The model under review builds one solid part; all positions refer to its coordinate system, in mm. Give positions to 0.01 mm unless a question says otherwise; leave off trailing zeros. Loops run counter-clockwise (first coordinate to the right, second up) from the corner with the lowest first, then second, coordinate; pieces in that order, holes last. Notation, with made-up numbers: M -5.75,-39 L 30.25,-39 A15 ccw 30.25,-35 Z; hole C -29,70 d3. An arc over 180 degrees is marked long. Put each result on its own line as item: value. Start each with the question number.
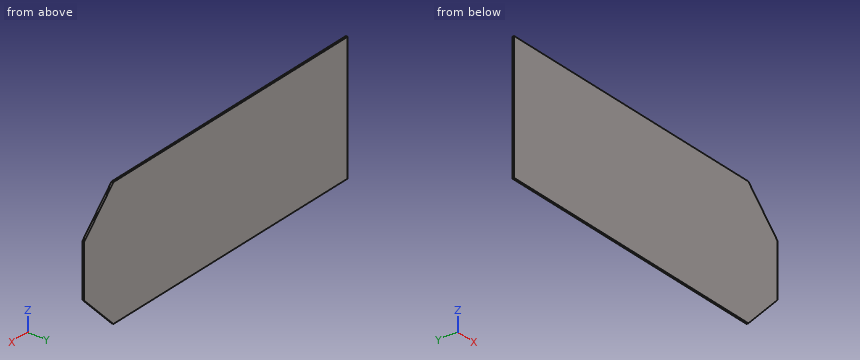
Autodesk Inventor part; units mm, degrees
ref_plane "YZ Plane" through (0, 0, 0) normal (1, 0, 0) x (0, 1, 0)
ref_plane "XZ Plane" through (0, 0, 0) normal (0, 1, 0) x (-1, 0, 0)
ref_plane "XY Plane" through (0, 0, 0) normal (0, 0, 1) x (1, 0, 0)
sketch "Sketch1" plane through (0, 0, 0) normal (0, 1, 0) x (-1, 0, 0)
  line L0 (-60.5593, 27.4889) -> (62.6411, -28.4339) construction
  line L1 (62.6424, 27.1286) -> (-64.3576, -27.8714) construction
  line L2 (-77.4954, -16.5) -> (-44.4954, -16.5) construction
  line L3 (-63.5, 27.7812) -> (63.5, 27.7812)
  line L4 (63.5, 27.7812) -> (63.5, -27.7812)
  line L5 (63.5, -27.7812) -> (-63.5, -27.7812)
  line L6 (-63.5, 27.7812) -> (63.5, -27.7812) construction
  line L7 (63.5, 27.7812) -> (-63.5, -27.7812) construction
  line L8 (-63.5, 11.5094) -> (63.5, 11.5094)
  line L9 (63.5, 11.5094) -> (63.5, -11.5094)
  line L10 (63.5, -11.5094) -> (-63.5, -11.5094)
  line L11 (-63.5, 11.5094) -> (63.5, -11.5094) construction
  line L12 (63.5, 11.5094) -> (-63.5, -11.5094) construction
  line L13 (-79.375, 11.5094) -> (-79.375, -11.5094)
  line L14 (-63.5, 27.7812) -> (-79.375, 11.5094)
  line L15 (-79.375, -11.5094) -> (-63.5, -27.7812)
  point P0 (0, 0)
  dimension "d1" = 55.5625
  dimension "d6" = 127
  dimension "d7" = 55.5625
  dimension "d8" = 127
  dimension "d9" = 23.0188
extrude "Extrusion1" add sketch "Sketch1" along normal mid plane 0.7874
properties part number "140x55mm-PCB"
(1) We need section A-A, the plane y = 0.2. Write out the cut boundary in (x, z) (3 decimals), plus the area to 3 significant figures.
(2) To check wall thickness, follow L1, parallel to X at y = -0.1, z = 24.5; L2, parallel to X at y = -0.25, z = -14; L3, parallel to Z at x = 72, y = 0.05. State the ranges of each line that lie inside material, in increasing order. Write a range as [from, to].
(3) We need section B-B, the plane z = 20.5. Write out the cut boundary in (x, y), plus the area to 3 significant figures.
(4) We need section C-C, the plane z = -17. Write out the cut boundary in (x, y), plus the area to 3 significant figures.
Check sheet entries:
1. outline: M -63.5,-27.781 L 63.5,-27.781 L 79.375,-11.509 L 79.375,11.509 L 63.5,27.781 L -63.5,27.781 Z
1. area: 7,680 mm²
2. L1: x = [-63.5, 66.7]
2. L2: x = [-63.5, 76.95]
2. L3: z = [-19.07, 19.07]
3. outline: M -63.5,-0.39 L 70.6,-0.39 L 70.6,0.39 L -63.5,0.39 Z
3. area: 106 mm²
4. outline: M -63.5,-0.39 L 74.02,-0.39 L 74.02,0.39 L -63.5,0.39 Z
4. area: 108 mm²
